CAD build for the part. Positions are in the model's coordinates, mm. A direction names the side the tool comes from. Round coordinates to 2 decimals unless told otherwise and drop trailing zeros. Loops run counter-clockwise (first coordinate to the right, second up) from the corner with the lowest first, then second, coordinate; pieces in that order, holes last.
from build123d import *

# Parameters (mm, degrees)
Y_KSEKLIK_EKSTR_ZYON1_DEPTH      = 9.5
Y_KSEKLIK_EKSTR_ZYON1_DEPTH_BACK = 9.5
IZIM7_R                          = 2.5
KES_EKSTR_ZYON2_DEPTH            = 19
Y_KSEKLIK_EKSTR_ZYON7_START      = 0.5
IZIM8_R                          = 4
IZIM8_R_2                        = 2.5
Y_KSEKLIK_EKSTR_ZYON7_DEPTH      = 0.5
IZIM9_R                          = 4
IZIM9_R_2                        = 2.5
Y_KSEKLIK_EKSTR_ZYON8_DEPTH      = 0.5
Y_KSEKLIK_EKSTR_ZYON9_DEPTH      = 19
Y_KSEKLIK_EKSTR_ZYON9_DEPTH_BACK = 19
IZIM10_R                         = 2.5
KES_EKSTR_ZYON4_DEPTH            = 9
KES_EKSTR_ZYON5_DEPTH            = 9
IZIM13_W                         = 5
IZIM13_H                         = 3
Y_KSEKLIK_EKSTR_ZYON10_DEPTH     = 5
IZIM14_R                         = 2
KES_EKSTR_ZYON6_DEPTH            = 5
RADYUS3_R                        = 0.5
Y_KSEKLIK_EKSTR_ZYON11_DEPTH     = 12
Y_KSEKLIK_EKSTR_ZYON12_DEPTH     = 19
Y_KSEKLIK_EKSTR_ZYON13_DEPTH     = 5
RADYUS4_R                        = 2
IZIM18_R                         = 5
Y_KSEKLIK_EKSTR_ZYON14_DEPTH     = 2
RADYUS5_R                        = 1
IZIM19_R                         = 0.5
Y_KSEKLIK_EKSTR_ZYON15_DEPTH     = 2
IZIM20_W                         = 3
IZIM20_H                         = 6
KES_EKSTR_ZYON7_DEPTH            = 1
IZIM21_W                         = 3
IZIM21_H                         = 6
KES_EKSTR_ZYON8_DEPTH            = 1
IZIM22_W                         = 1
IZIM22_H                         = 6
Y_KSEKLIK_EKSTR_ZYON17_DEPTH     = 3
IZIM23_W                         = 6
IZIM23_H                         = 1
Y_KSEKLIK_EKSTR_ZYON18_DEPTH     = 2
IZIM24_W                         = 1
IZIM24_H                         = 6
Y_KSEKLIK_EKSTR_ZYON19_DEPTH     = 3
IZIM25_W                         = 6
IZIM25_H                         = 1
Y_KSEKLIK_EKSTR_ZYON20_DEPTH     = 2


with BuildPart() as part:
    # Çizim1 → Yükseklik-Ekstrüzyon1 (new, two sides: drawn at the far end of the back side and taken through both)
    with BuildSketch(Plane(origin=(0, 0, 0), x_dir=(1, 0, 0), z_dir=(0, 1, 0)).offset(-Y_KSEKLIK_EKSTR_ZYON1_DEPTH_BACK)):
        with BuildLine():
            Line((-18.5, 11), (15.5, 11))
            ThreePointArc((15.5, 11), (17.621320344, 10.121320344), (18.5, 8))
            Line((18.5, 8), (18.5, -8))
            ThreePointArc((18.5, -8), (17.621320344, -10.121320344), (15.5, -11))
            Line((15.5, -11), (-18.5, -11))
            Line((-18.5, -11), (-18.5, 11))
        make_face()
    extrude(amount=Y_KSEKLIK_EKSTR_ZYON1_DEPTH + Y_KSEKLIK_EKSTR_ZYON1_DEPTH_BACK)

    # Çizim7 → Kes-Ekstrüzyon2 (cut)
    with BuildSketch(Plane(origin=(0, 9.5, 0), x_dir=(1, 0, 0), z_dir=(0, 1, 0))):
        with Locations(Location((7.5, 0, 0), (0, 0, 270))):
            Circle(IZIM7_R)
    extrude(amount=-KES_EKSTR_ZYON2_DEPTH, mode=Mode.SUBTRACT)

    # Çizim8 → Yükseklik-Ekstrüzyon7 (add)
    with BuildSketch(Plane(origin=(0, 9.5, 0), x_dir=(1, 0, 0), z_dir=(0, 1, 0)).offset(Y_KSEKLIK_EKSTR_ZYON7_START)):
        with Locations(Location((7.5, 0, 0), (0, 0, 270))):
            Circle(IZIM8_R)
        with Locations(Location((7.5, 0, 0), (0, 0, 270))):
            Circle(IZIM8_R_2, mode=Mode.SUBTRACT)
    extrude(amount=-Y_KSEKLIK_EKSTR_ZYON7_DEPTH)

    # Çizim9 → Yükseklik-Ekstrüzyon8 (add)
    with BuildSketch(Plane.XZ.offset(9.5)):
        with Locations(Location((7.5, 0, 0), (0, 0, 90))):
            Circle(IZIM9_R)
        with Locations(Location((7.5, 0, 0), (0, 0, 90))):
            Circle(IZIM9_R_2, mode=Mode.SUBTRACT)
    extrude(amount=Y_KSEKLIK_EKSTR_ZYON8_DEPTH)

    # Çizim10 → Yükseklik-Ekstrüzyon9 (add, two sides: drawn at the far end of the back side and taken through both)
    with BuildSketch(Plane(origin=(0, 0, 0), x_dir=(1, 0, 0), z_dir=(0, 1, 0)).offset(-Y_KSEKLIK_EKSTR_ZYON9_DEPTH_BACK)):
        with Locations(Location((7.5, 0, 0), (0, 0, 270))):
            Circle(IZIM10_R)
    extrude(amount=Y_KSEKLIK_EKSTR_ZYON9_DEPTH + Y_KSEKLIK_EKSTR_ZYON9_DEPTH_BACK)

    # Çizim11 → Kes-Ekstrüzyon4 (cut)
    with BuildSketch(Plane(origin=(0, 19, 0), x_dir=(1, 0, 0), z_dir=(0, 1, 0))):
        with BuildLine():
            Line((5.5, 1.5), (5.5, -1.5))
            ThreePointArc((5.5, -1.5), (5, 0), (5.5, 1.5))
        make_face()
        with BuildLine():
            Line((9.5, 1.5), (9.5, -1.5))
            ThreePointArc((9.5, -1.5), (10, 0), (9.5, 1.5))
        make_face()
    extrude(amount=-KES_EKSTR_ZYON4_DEPTH, mode=Mode.SUBTRACT)

    # Çizim12 → Kes-Ekstrüzyon5 (cut)
    with BuildSketch(Plane.XZ.offset(19)):
        with BuildLine():
            Line((5.5, 1.5), (5.5, -1.5))
            ThreePointArc((5.5, -1.5), (5, 0), (5.5, 1.5))
        make_face()
        with BuildLine():
            Line((9.5, 1.5), (9.5, -1.5))
            ThreePointArc((9.5, -1.5), (10, 0), (9.5, 1.5))
        make_face()
    extrude(amount=-KES_EKSTR_ZYON5_DEPTH, mode=Mode.SUBTRACT)

    # Çizim13 → Yükseklik-Ekstrüzyon10 (add)
    with BuildSketch(Plane(origin=(18.5, 0, 0), x_dir=(0, 0, -1), z_dir=(1, 0, 0))):
        Rectangle(IZIM13_W, IZIM13_H)
    extrude(amount=Y_KSEKLIK_EKSTR_ZYON10_DEPTH)

    # Çizim14 → Kes-Ekstrüzyon6 (cut)
    with BuildSketch(Plane.XZ.offset(1.5)):
        with Locations(Location((21, 0, 0), (0, 0, 270))):
            Circle(IZIM14_R)
    extrude(amount=-KES_EKSTR_ZYON6_DEPTH, mode=Mode.SUBTRACT)

    # Radyus3
    radyus3_edges = [part.edges().sort_by_distance(p)[0] for p in [
        (23.5, 0, -2.5),
        (23.5, 0, 2.5),
    ]]
    fillet(radyus3_edges, radius=RADYUS3_R)

    # Çizim15 → Yükseklik-Ekstrüzyon11 (add)
    with BuildSketch(Plane.ZY.offset(18.5)):
        with BuildLine():
            Line((5.545268253, 9.5), (-5.545268253, 9.5))
            ThreePointArc((-5.545268253, 9.5), (-11, 0), (-5.545268253, -9.5))
            Line((-5.545268253, -9.5), (5.545268253, -9.5))
            ThreePointArc((5.545268253, -9.5), (10.965120348, -0.875291809), (6.982120022, 8.5))
            ThreePointArc((6.982120022, 8.5), (6.283618722, 9.028628675), (5.545268253, 9.5))
        make_face()
        with BuildLine():
            ThreePointArc((-5.267826876, -8.5), (-10, 0), (-5.267826876, 8.5))
            Line((-5.267826876, 8.5), (5.267826876, 8.5))
            ThreePointArc((5.267826876, 8.5), (10, 0), (5.267826876, -8.5))
            Line((5.267826876, -8.5), (-5.267826876, -8.5))
        make_face(mode=Mode.SUBTRACT)
    extrude(amount=Y_KSEKLIK_EKSTR_ZYON11_DEPTH)

    # Çizim16 → Yükseklik-Ekstrüzyon12 (add)
    with BuildSketch(Plane.ZY.offset(18.5)):
        with BuildLine():
            Line((-5.267826876, 8.5), (5.267826876, 8.5))
            ThreePointArc((5.267826876, 8.5), (10, 0), (5.267826876, -8.5))
            Line((5.267826876, -8.5), (-5.267826876, -8.5))
            ThreePointArc((-5.267826876, -8.5), (-10, 0), (-5.267826876, 8.5))
        make_face()
    extrude(amount=Y_KSEKLIK_EKSTR_ZYON12_DEPTH)

    # Çizim17 → Yükseklik-Ekstrüzyon13 (add)
    with BuildSketch(Plane.ZY.offset(37.5)):
        with BuildLine():
            Line((-5.267826876, 8.5), (5.267826876, 8.5))
            ThreePointArc((5.267826876, 8.5), (10, 0), (5.267826876, -8.5))
            Line((5.267826876, -8.5), (-5.267826876, -8.5))
            ThreePointArc((-5.267826876, -8.5), (-10, 0), (-5.267826876, 8.5))
        make_face()
    extrude(amount=Y_KSEKLIK_EKSTR_ZYON13_DEPTH)

    # Radyus4
    # the kernel refuses this fillet: 2 mm, written as the material it takes off along each edge
    with BuildSketch(Plane(origin=(-42.5, 0, 0), x_dir=(0, -0.9985166114955222, -0.05444792528187306), z_dir=(0, -0.05444792528187306, 0.9985166114955222))) as radyus4_piece_1:
        with BuildLine():
            CenterArc((10 - RADYUS4_R, RADYUS4_R), RADYUS4_R, 270, 90)
            Line((10, RADYUS4_R), (10, 0))
            Line((10, 0), (10 - RADYUS4_R, 0))
        make_face()
    revolve(axis=Axis((-42.5, 0, 0), (1, 0, 0)), revolution_arc=173.757640436, mode=Mode.SUBTRACT)
    with BuildSketch(Plane(origin=(-42.5, -8.5, 10.267826876), x_dir=(1, 0, 0), z_dir=(0, 0, -1))) as radyus4_piece_2:
        with BuildLine():
            CenterArc((RADYUS4_R, -RADYUS4_R), RADYUS4_R, 90, 90)
            Line((0, -RADYUS4_R), (0, 0))
            Line((0, 0), (RADYUS4_R, 0))
        make_face()
    extrude(amount=20.535653753, mode=Mode.SUBTRACT)
    with BuildSketch(Plane(origin=(-42.5, 0, 0), x_dir=(0, 0.9985166114955222, 0.05444792528187289), z_dir=(0, 0.05444792528187289, -0.9985166114955222))) as radyus4_piece_3:
        with BuildLine():
            CenterArc((10 - RADYUS4_R, RADYUS4_R), RADYUS4_R, 270, 90)
            Line((10, RADYUS4_R), (10, 0))
            Line((10, 0), (10 - RADYUS4_R, 0))
        make_face()
    revolve(axis=Axis((-42.5, 0, 0), (1, 0, 0)), revolution_arc=173.757640436, mode=Mode.SUBTRACT)
    with BuildSketch(Plane(origin=(-42.5, 8.5, -10.267826876), x_dir=(0, -1, 0), z_dir=(0, 0, 1))) as radyus4_piece_4:
        with BuildLine():
            CenterArc((RADYUS4_R, RADYUS4_R), RADYUS4_R, 180, 90)
            Line((0, RADYUS4_R), (0, 0))
            Line((0, 0), (RADYUS4_R, 0))
        make_face()
    extrude(amount=20.535653753, mode=Mode.SUBTRACT)

    # Çizim18 → Yükseklik-Ekstrüzyon14 (add)
    with BuildSketch(Plane.ZY.offset(42.5)):
        Circle(IZIM18_R)
    extrude(amount=Y_KSEKLIK_EKSTR_ZYON14_DEPTH)

    # Radyus5
    radyus5_edges = [part.edges().sort_by_distance(p)[0] for p in [
        (-44.5, 0, -5),
    ]]
    fillet(radyus5_edges, radius=RADYUS5_R)

    # Çizim19 → Yükseklik-Ekstrüzyon15 (add)
    with BuildSketch(Plane.ZY.offset(44.5)):
        Circle(IZIM19_R)
    extrude(amount=Y_KSEKLIK_EKSTR_ZYON15_DEPTH)

    # Çizim20 → Kes-Ekstrüzyon7 (cut)
    with BuildSketch(Plane(origin=(0, 9.5, 0), x_dir=(1, 0, 0), z_dir=(0, 1, 0))):
        with Locations((-24, 0)):
            Rectangle(IZIM20_W, IZIM20_H)
    extrude(amount=-KES_EKSTR_ZYON7_DEPTH, mode=Mode.SUBTRACT)

    # Çizim21 → Kes-Ekstrüzyon8 (cut)
    with BuildSketch(Plane.XZ.offset(9.5)):
        with Locations((-24, 0)):
            Rectangle(IZIM21_W, IZIM21_H)
    extrude(amount=-KES_EKSTR_ZYON8_DEPTH, mode=Mode.SUBTRACT)

    # Çizim22 → Yükseklik-Ekstrüzyon17 (add)
    with BuildSketch(Plane.XZ.offset(9.5)):
        with Locations((-26, 0)):
            Rectangle(IZIM22_W, IZIM22_H)
    extrude(amount=Y_KSEKLIK_EKSTR_ZYON17_DEPTH)

    # Çizim23 → Yükseklik-Ekstrüzyon18 (add)
    with BuildSketch(Plane(origin=(-25.5, 0, 0), x_dir=(0, 0, -1), z_dir=(1, 0, 0))):
        with Locations((0, -12)):
            Rectangle(IZIM23_W, IZIM23_H)
    extrude(amount=Y_KSEKLIK_EKSTR_ZYON18_DEPTH)

    # Çizim24 → Yükseklik-Ekstrüzyon19 (add)
    with BuildSketch(Plane(origin=(0, 9.5, 0), x_dir=(1, 0, 0), z_dir=(0, 1, 0))):
        with Locations((-26, 0)):
            Rectangle(IZIM24_W, IZIM24_H)
    extrude(amount=Y_KSEKLIK_EKSTR_ZYON19_DEPTH)

    # Çizim25 → Yükseklik-Ekstrüzyon20 (add)
    with BuildSketch(Plane(origin=(-25.5, 0, 0), x_dir=(0, 0, -1), z_dir=(1, 0, 0))):
        with Locations((0, 12)):
            Rectangle(IZIM25_W, IZIM25_H)
    extrude(amount=Y_KSEKLIK_EKSTR_ZYON20_DEPTH)


solid = part.part
Item 1: 3-axis set-ups, long thin cutter, end or side, ignore diameter. For faces 1 (the cylindrical face through (7.5, -14.6, 2.5)), 2 (the flat face through (9.5, 15, 0)), 3 (the flat face through (5.5, -15, 0)), 4 (the flat face through (5.5, 15, 0)), 5 (the flat face through (-25.5, -10, 0)): which of +Z, -Z, +X, -X, +Y, -Y reach the whole face in a straight line?
Verdict:
face 1: +Z, -Y
face 2: +Z, -Z, +X, +Y
face 3: +Z, -Z, -Y
face 4: +Z, -Z, +Y
face 5: none
Item 2: Cut at C-C (x = -37.5). List the corners of the cut face in (y, z), plus the area to 3 significant figures.
Verdict:
outline: (-8.5, -5.27) arc R10 ccw to (8.5, -5.27) - (8.5, 5.27) arc R10 ccw to (-8.5, 5.27) - close
area: 293 mm2
Item 3: Cut at D-D (x = -13.5). List the corners of the cut face in (y, z).
Verdict:
outline: (-9.5, -11) - (9.5, -11) - (9.5, 11) - (-9.5, 11) - close
Item 4: Wall check: L1, parallel to X at y = -0.9, z = 0; L2, parallel to Y at x = 3.5, z = 2.25; L3, parallel to X at y = -2, z = 2.5. Give the ranges that are in metal, low to high.
Verdict:
L1: x = -44.5 to 19, 23 to 23.5
L2: y = -9.5 to 9.5
L3: x = -44.5 to 18.5
Item 5: Cut at A-A (x = 21). List the corners of the cut face in (y, z), plus the area to 3 significant figures.
Verdict:
outline: (-1.5, -2.5) - (1.5, -2.5) - (1.5, -2) - (-1.5, -2) - close; (-1.5, 2) - (1.5, 2) - (1.5, 2.5) - (-1.5, 2.5) - close
area: 3.00 mm2
Item 6: Mould opens along Z. For faces 6 (the flat face through (10, -10, 0)), 7 (the flat face through (-25.5, 10, 0)), 8 (the cylindrical face through (-24, 0, -11)), 9 (the flat face through (-26, -11, 3)) say: released by +Z, released by -Z, zero draft, split by the parting line, or undercut.
Verdict:
face 6: zero draft
face 7: undercut
face 8: released by -Z
face 9: released by +Z
Item 7: Cut at B-B (x = 7.5). List the corners of the cut face in (y, z).
Verdict:
outline: (-19, -2.5) - (-10, -2.5) - (-10, -4) - (-9.5, -4) - (-9.5, -11) - (9.5, -11) - (9.5, -4) - (10, -4) - (10, -2.5) - (19, -2.5) - (19, 2.5) - (10, 2.5) - (10, 4) - (9.5, 4) - (9.5, 11) - (-9.5, 11) - (-9.5, 4) - (-10, 4) - (-10, 2.5) - (-19, 2.5) - close
Item 8: Flat gauge pins, fed straight in: P1, Ø0.5, axis at x = -24, y = -9, coming from the +Z side; P2, Ø1.6, axis at y = 2.5, z = 8, coming from the -X side; P3, Ø5, axis at x = 8, z = -3.5, coming from the -Y side; P4, Ø1, axis at x = -24, z = 0, coming from the -Y side. Where does each tip first touch, or does it go through?
Verdict:
P1: stops at z = 6.67
P2: stops at x = -42.5
P3: stops at y = -19
P4: stops at y = -12.5
